Autodesk Inventor part; units mm, degrees
ref_plane "YZ Plane" through (0, 0, 0) normal (1, 0, 0) x (0, 1, 0)
ref_plane "XZ Plane" through (0, 0, 0) normal (0, 1, 0) x (-1, 0, 0)
ref_plane "XY Plane" through (0, 0, 0) normal (0, 0, 1) x (1, 0, 0)
sketch "Skizze1" plane through (0, 0, 0) normal (0, 0, 1) x (1, 0, 0)
  circle A0 centre (0, 0) radius 2
  dimension "Breite" = 4
extrude "Extrusion1" add sketch "Skizze1" along normal blind 25
chamfer "Fase1" distance 0.5 angle 45 1 edges at (-2, 0, 0)
chamfer "Fase2" distance 0.5 angle 45 1 edges at (-2, 0, 25) measured on face at (1.9741, -0.3208, 16.8333)
properties part number "Stift"
Work out the finished part from the listing and answer in its coordinate system (mm). Give positions to 0.01 mm unless a question says otherwise; leave off trailing zeros. Order: outer loops, then holes, each group sorted by start corner. A loop starts at its lowest first (then second) coordinate and runs counter-clockwise, first axis right, second up. Notation, with made-up numbers: M 19.25,43.25 L 49.25,43.25 A26 ccw 49.25,71.25 Z; hole C -34,43.5 d9. An arc over 180 degrees is marked long. Return JSON: item names as keys, results as strings.
Q1. Find the intervals of material crossed by line 1 along Y through (x, z) = (-1.55, 7); line 2 along Y through (x, z) = (-1.8, 18.5); line 3 along Z through (x, y) = (0.55, 1.4), in increasing order. Write a range as [from, to].
Answer below:
{"line 1": "y = [-1.26, 1.26]", "line 2": "y = [-0.87, 0.87]", "line 3": "z = [0, 25]"}
Q2. This flat-tipped pin is pushed along its axis until it touches: pin 1 (1 mm diameter, centred on x = 1, z = 17.5, fed in from -Y). Where does it stop, or does it pass through?
Answer below:
{"pin 1": "stops at y = -1.94"}
Q3. Find section A-A, the plane z = 10.5. Write down the section's boundary in (x, y).
Answer below:
{"outline": "C 0,0 d4"}
